Input: part model. Units: mm. Frame: model coordinates. Face numbers are marked on the shaded views. A direction names the side the tool comes from. Give positions to 0.01 mm unless a question says otherwise; leave off trailing zeros. Loops run counter-clockwise (first coordinate to the right, second up) from the corner with the lowest first, then second, coordinate; pieces in that order, holes last. Notation, with made-up numbers: (31.25, 42) -> (74.25, 42) arc R10 cw to (74.25, 46) -> close; hole circle Ø6 at (15.5, -33.75). An arc over 180 degrees is marked (long way). Use CSV: the item, a comma, the result in double quotes.
```python
from build123d import *

# Parameters (mm, degrees)
SKETCH1_R           = 90
BOSS_EXTRUDE1_DEPTH = 75
SKETCH2_R           = 87.5
CUT_EXTRUDE1_DEPTH  = 70
SKETCH3_R           = 32.5
BOSS_EXTRUDE2_DEPTH = 70
SKETCH4_W           = 180
SKETCH4_H           = 66
CUT_EXTRUDE2_DEPTH  = 75
SKETCH5_W           = 175
SKETCH5_H           = 61.187525855
CUT_EXTRUDE3_DEPTH  = 75
SKETCH6_W           = 179.999459639
SKETCH6_H           = 83.811872958
CUT_EXTRUDE4_DEPTH  = 75
SKETCH8_W           = 180
SKETCH8_H           = 71
BOSS_EXTRUDE5_DEPTH = 75
BOSS_EXTRUDE6_REACH = 182
SKETCH10_W          = 20
SKETCH10_H          = 75
BOSS_EXTRUDE7_REACH = 182
SKETCH11_W          = 20
SKETCH11_H          = 75
SKETCH12_W          = 175
SKETCH12_H          = 65
CUT_EXTRUDE5_DEPTH  = 70
CUT_EXTRUDE6_DEPTH  = 70
CUT_EXTRUDE7_DEPTH  = 10
BOSS_EXTRUDE8_DEPTH = 50
CUT_EXTRUDE8_DEPTH  = 50


with BuildPart() as part:
    # Sketch1 → Boss-Extrude1 (new body)
    with BuildSketch(Plane(origin=(0, 0, 0), x_dir=(1, 0, 0), z_dir=(0, 1, 0))):
        Circle(SKETCH1_R)
    extrude(amount=BOSS_EXTRUDE1_DEPTH)

    # Sketch2 → Cut-Extrude1 (cut)
    with BuildSketch(Plane(origin=(0, 75, 0), x_dir=(1, 0, 0), z_dir=(0, 1, 0))):
        Circle(SKETCH2_R)
    extrude(amount=-CUT_EXTRUDE1_DEPTH, mode=Mode.SUBTRACT)

    # Sketch3 → Boss-Extrude2 (add)
    with BuildSketch(Plane(origin=(0, 5, 0), x_dir=(1, 0, 0), z_dir=(0, 1, 0))):
        Circle(SKETCH3_R)
    extrude(amount=BOSS_EXTRUDE2_DEPTH)

    # Sketch4 → Cut-Extrude2 (cut)
    with BuildSketch(Plane(origin=(0, 75, 0), x_dir=(1, 0, 0), z_dir=(0, 1, 0))):
        with Locations((0, -65.5)):
            Rectangle(SKETCH4_W, SKETCH4_H)
    extrude(amount=-CUT_EXTRUDE2_DEPTH, mode=Mode.SUBTRACT)

    # Sketch5 → Cut-Extrude3 (cut)
    with BuildSketch(Plane(origin=(0, 75, 0), x_dir=(1, 0, 0), z_dir=(0, 1, 0))):
        with Locations((-0.249643874, -50.593762928)):
            Rectangle(SKETCH5_W, SKETCH5_H)
    extrude(amount=-CUT_EXTRUDE3_DEPTH, mode=Mode.SUBTRACT)

    # Sketch6 → Cut-Extrude4 (cut)
    with BuildSketch(Plane(origin=(0, 75, 0), x_dir=(1, 0, 0), z_dir=(0, 1, 0))):
        with Locations((0.00027018, -61.905936479)):
            Rectangle(SKETCH6_W, SKETCH6_H)
    extrude(amount=-CUT_EXTRUDE4_DEPTH, mode=Mode.SUBTRACT)

    # Sketch8 → Boss-Extrude5 (add)
    with BuildSketch(Plane(origin=(0, 75, 0), x_dir=(1, 0, 0), z_dir=(0, 1, 0))):
        with Locations((0, -55.5)):
            Rectangle(SKETCH8_W, SKETCH8_H)
    extrude(amount=-BOSS_EXTRUDE5_DEPTH)

    # Sketch10 → Boss-Extrude6 (add, up to next)
    with BuildSketch(Plane.ZY.offset(90), mode=Mode.PRIVATE) as boss_extrude6_sk1:
        with Locations((10, 37.5)):
            Rectangle(SKETCH10_W, SKETCH10_H)
    boss_extrude6_tool1 = extrude(boss_extrude6_sk1.sketch, amount=-BOSS_EXTRUDE6_REACH, mode=Mode.PRIVATE) - part.part
    add(boss_extrude6_tool1.solids().sort_by_distance((-90, 37.5, 10))[0])

    # Sketch11 → Boss-Extrude7 (add, up to next)
    with BuildSketch(Plane(origin=(90, 0, 0), x_dir=(0, 0, -1), z_dir=(1, 0, 0)), mode=Mode.PRIVATE) as boss_extrude7_sk1:
        with Locations((-10, 37.5)):
            Rectangle(SKETCH11_W, SKETCH11_H)
    boss_extrude7_tool1 = extrude(boss_extrude7_sk1.sketch, amount=-BOSS_EXTRUDE7_REACH, mode=Mode.PRIVATE) - part.part
    add(boss_extrude7_tool1.solids().sort_by_distance((90, 37.5, 10))[0])

    # Sketch12 → Cut-Extrude5 (cut)
    with BuildSketch(Plane(origin=(0, 75, 0), x_dir=(1, 0, 0), z_dir=(0, 1, 0))):
        with Locations((0, -55.5)):
            Rectangle(SKETCH12_W, SKETCH12_H)
    extrude(amount=-CUT_EXTRUDE5_DEPTH, mode=Mode.SUBTRACT)

    # Sketch13 → Cut-Extrude6 (cut)
    with BuildSketch(Plane.ZY.offset(-87.5)):
        with BuildLine():
            Line((50.5, 27.25), (58.5, 27.25))
            ThreePointArc((58.5, 27.25), (60.25, 25.5), (58.5, 23.75))
            Line((58.5, 23.75), (50.5, 23.75))
            ThreePointArc((50.5, 23.75), (48.75, 25.5), (50.5, 27.25))
        make_face()
    extrude(amount=-CUT_EXTRUDE6_DEPTH, mode=Mode.SUBTRACT)

    # Sketch14 → Cut-Extrude7 (cut)
    with BuildSketch(Plane.XY.offset(91)):
        with BuildLine():
            Line((41.5, 21.25), (31.5, 21.25))
            ThreePointArc((31.5, 21.25), (29.5, 23.25), (31.5, 25.25))
            Line((31.5, 25.25), (41.5, 25.25))
            ThreePointArc((41.5, 25.25), (43.5, 23.25), (41.5, 21.25))
        make_face()
    extrude(amount=-CUT_EXTRUDE7_DEPTH, mode=Mode.SUBTRACT)

    # Sketch15 → Boss-Extrude8 (add)
    with BuildSketch(Plane(origin=(0, 0, 20), x_dir=(-1, 0, 0), z_dir=(0, 0, -1))):
        Polygon((55.400501051, 5), (57.12123036, 7.457456133), (56.12123036, 7.457456133), (54.400501051, 5), align=None)
        Polygon((73.679771742, 7.457456133), (74.679771742, 7.457456133), (76.400501051, 5), (75.400501051, 5), align=None)
    extrude(amount=BOSS_EXTRUDE8_DEPTH)

    # Sketch17 → Cut-Extrude8 (cut)
    with BuildSketch(Plane.ZY.offset(90)):
        with BuildLine():
            Line((84, 69), (84, 54))
            ThreePointArc((84, 54), (80.5, 50.5), (77, 54))
            Line((77, 54), (77, 69))
            ThreePointArc((77, 69), (80.5, 72.5), (84, 69))
        make_face()
    extrude(amount=-CUT_EXTRUDE8_DEPTH, mode=Mode.SUBTRACT)


solid = part.part
```
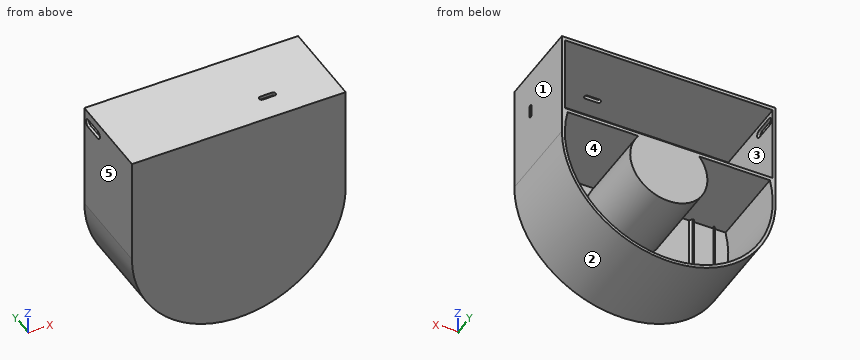
1) Section query C-C (z = -25). Return loops of the section in (x, y).
From the geometry:
outline,"(-86.46, 0) -> (86.46, 0) -> (86.46, 75) -> (83.85, 75) -> (83.85, 5) -> (20.77, 5) -> (20.77, 75) -> (-20.77, 75) -> (-20.77, 5) -> (-54.4, 5) -> (-56.12, 7.46) -> (-57.12, 7.46) -> (-55.4, 5) -> (-75.4, 5) -> (-73.68, 7.46) -> (-74.68, 7.46) -> (-76.4, 5) -> (-83.85, 5) -> (-83.85, 75) -> (-86.46, 75) -> close"
2) Section query A-A (y = 16). Return loops of the section in (x, z), then the cut area to 3 significant figures.
From the geometry:
outline,"(-90, 0) arc R90 ccw to (90, 0) -> (90, 91) -> (-90, 91) -> close; hole (-87.5, 23) -> (87.5, 23) -> (87.5, 88) -> (-87.5, 88) -> close; hole (-85.18, 20) arc R87.5 ccw (long way) to (85.18, 20) -> (25.62, 20) arc R32.5 cw (long way) to (-25.62, 20) -> close"
area,"5,100 mm^2"
3) Reachability of the marked faces 4 and 5 from +Z, -Z, +X, -X, +Y, -Y: full face, straight path, thin tool, end or side. Return the list, or none.
From the geometry:
face 4,"+Y"
face 5,"+Z, -Z, -X, +Y, -Y"
4) Section query D-D (x = -37). Return loops of the section in (y, z), then the cut area to 3 significant figures.
From the geometry:
outline,"(0, -82.04) -> (75, -82.04) -> (75, -79.29) -> (5, -79.29) -> (5, 20) -> (75, 20) -> (75, 23) -> (5, 23) -> (5, 88) -> (75, 88) -> (75, 91) -> (0, 91) -> close"
area,"1,480 mm^2"
5) Mould query, pull axis Z, two halves, no side actions, for the marked faces 1, 2 and 3. Classes: pulls with the +Z half, pulls with the -Z half, needs draft (parallel to the pull), parting line crosses it, or undercut.
From the geometry:
face 1,"needs draft"
face 2,"pulls with the -Z half"
face 3,"undercut"
6) Ray query, line 1 (X direction, y = 42, z = 0); line 2 (Z direction, x = 0, y = 38); line 3 (X direction, y = 14.5, z = 24.5). Return the intervals inside material, ascending.
From the geometry:
line 1,"x = -90 to -87.5, -32.5 to 32.5, 87.5 to 90"
line 2,"z = -90 to -87.5, -32.5 to 23, 88 to 91"
line 3,"x = -90 to -87.5, 87.5 to 90"
7) Section query B-B (x = 39). Return loops of the section in (y, z).
From the geometry:
outline,"(0, -81.11) -> (75, -81.11) -> (75, -78.33) -> (5, -78.33) -> (5, 20) -> (75, 20) -> (75, 23) -> (5, 23) -> (5, 88) -> (21.25, 88) -> (21.25, 91) -> (0, 91) -> close; (25.25, 88) -> (75, 88) -> (75, 91) -> (25.25, 91) -> close"
8) Contact query for flat-ended pins moving along their axis: pin 1 (2.5 mm diameter, centred on x = -55.5, y = 6, fed in from -Z); pin 2 (18 mm diameter, centred on x = -60.5, y = 52, fed in from -Z); pin 3 (0.7 mm diameter, centred on x = -75.5, y = 6.5, fed in from -Z). Output: stop coordinate, or through.
From the geometry:
pin 1,"stops at z = -71.81"
pin 2,"stops at z = -73.81"
pin 3,"stops at z = -49.52"
